Study the drawing (mm; zero at the part's minimum x, y, z) and answer. A direction names the side the tool comes from. Coordinates: 2 decimals unless noted, no trailing zeros. Loops run counter-clockwise (first coordinate to the right, second up) from the corner with the lowest first, then second, coordinate; pieces in that order, holes last. Notation, with made-up numbers: (48.5, 9.5) - (89.5, 9.5) arc R17 ccw to (89.5, 39.5) - close; hole circle Ø3 at (86, -37.75). An arc over 180 degrees is marked (long way). One line per item, written item: value. Start each with the question number.
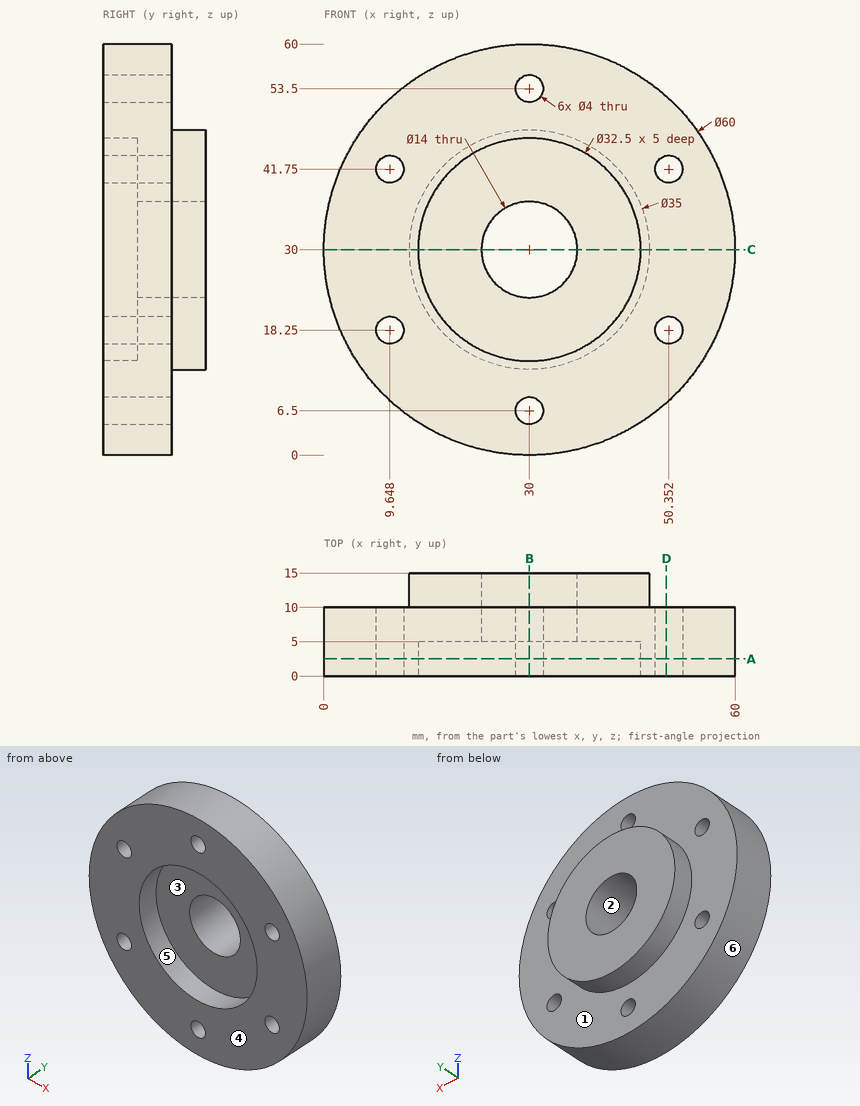
1) Section A-A, the plane y = 2.5 is taken. Determine the outline of the cut face in (x, z), and give its area (3 significant figures).
2) Section C-C, the plane z = 30 is taken. Determine the outline of the cut face in (x, y).
3) Straight lines are drawn through the part: L1, parallel to Z at x = 30, y = 3.1; L2, parallel to Z at x = 30, y = 5.25; L3, parallel to X at y = 7.75, z = 17 (1 decimal). For each, find the intervals that lie inside material, in ascending order.
4) Section D-D, the plane x = 50 is taken. Determine the outline of the cut face in (y, z).
5) Determine the mould class of the marked faces 4, 5 and 6 for opening direction X: released by +X, released by -X, zero draft, split by the parting line, or undercut.
6) Section B-B, the plane x = 30 is taken. Determine the outline of the cut face in (y, z).
7) For the marked faces 1, 2 and 3, determine the directions among +Z, -Z, +X, -X, +Y, -Y from which every point of the face is accessible in a straight line to the end or side of a thin tool.
8) Flat-ended cylindrical pins translate along their axes: P1, Ø1.5, axis at x = 12.5, y = 6.5, coming from the +Z side; P2, Ø6.5, axis at x = 9.65, z = 41.75, coming from the +Y side; P3, Ø19.5, axis at x = 30, z = 30, coming from the -Y side; P4, Ø10, axis at x = 11, z = 54, coming from the -Y side. Find the tip coordinate at first contact, or state that the pin passes through.
Answer below:
1. outline: circle Ø60 at (30, 30); hole circle Ø4 at (9.65, 18.25); hole circle Ø4 at (9.65, 41.75); hole circle Ø32.5 at (30, 30); hole circle Ø4 at (30, 6.5); hole circle Ø4 at (30, 53.5); hole circle Ø4 at (50.35, 18.25); hole circle Ø4 at (50.35, 41.75)
1. area: 1,920 mm2
2. outline: (0, 0) - (13.75, 0) - (13.75, 5) - (23, 5) - (23, 15) - (12.5, 15) - (12.5, 10) - (0, 10) - close; (37, 5) - (46.25, 5) - (46.25, 0) - (60, 0) - (60, 10) - (47.5, 10) - (47.5, 15) - (37, 15) - close
3. L1: 0 to 4.5, 8.5 to 13.75, 46.25 to 51.5, 55.5 to 60
3. L2: 0 to 4.5, 8.5 to 23, 37 to 51.5, 55.5 to 60
3. L3: 3 to 8.1, 11.2 to 48.8, 51.9 to 57
4. outline: (0, 7.64) - (10, 7.64) - (10, 16.28) - (0, 16.28) - close; (0, 20.22) - (10, 20.22) - (10, 39.78) - (0, 39.78) - close; (0, 43.72) - (10, 43.72) - (10, 52.36) - (0, 52.36) - close
5. face 4: zero draft
5. face 5: undercut
5. face 6: split by the parting line
6. outline: (0, 0) - (10, 0) - (10, 4.5) - (0, 4.5) - close; (0, 8.5) - (10, 8.5) - (10, 12.5) - (15, 12.5) - (15, 23) - (5, 23) - (5, 13.75) - (0, 13.75) - close; (0, 46.25) - (5, 46.25) - (5, 37) - (15, 37) - (15, 47.5) - (10, 47.5) - (10, 51.5) - (0, 51.5) - close; (0, 55.5) - (10, 55.5) - (10, 60) - (0, 60) - close
7. face 1: +Y
7. face 2: +Y, -Y
7. face 3: -Y
8. P1: z = 54.89
8. P2: y = 10
8. P3: y = 5
8. P4: y = 0
